Work out the finished part from the listing and answer in its coordinate system (mm). A direction names the side the tool comes from. Round coordinates to 2 decimals unless told otherwise and drop trailing zeros. Loops run counter-clockwise (first coordinate to the right, second up) from the corner with the lowest first, then second, coordinate; pieces in that order, holes last. Notation, with made-up numbers: (49, 61.25) -> (92, 61.25) arc R24 ccw to (92, 71.25) -> close; hole circle Ø6 at (42.25, 78). An arc over 180 degrees is marked (long way). Use CSV: the item, a comma, the result in double quotes. Start each with the question number.
from build123d import *

# Parameters (mm, degrees)
F0_R     = 45
F1_DEPTH = 8
F2_R     = 5
F3_W     = 23
F3_H     = 12.6
F4_DEPTH = 16.5
F5_T     = 2.5


with BuildPart() as f1:
    # F0 (on Top) → F1 (new body)
    with BuildSketch(Plane.XY):
        Circle(F0_R)
    extrude(amount=F1_DEPTH)

    # F2
    f2_edges = [f1.edges().sort_by_distance(p)[0] for p in [
        (-45, 0, 8),
    ]]
    fillet(f2_edges, radius=F2_R)

    # F3 (on Top) → F4 (join)
    with BuildSketch(Plane.XY):
        Rectangle(F3_W, F3_H)
    extrude(amount=F4_DEPTH)

    # F5
    f5_openings = [f1.faces().sort_by_distance(p)[0] for p in [
        (0, 0, 16.5),
    ]]
    offset(amount=F5_T, openings=f5_openings, kind=Kind.INTERSECTION)


solid = f1.part
Q1. For a pull along X with two mould halves and no side action, classify faces 6 (the flat face through (0, 8.8, 13)), 7 (the flat face through (11.5, 0, 12)), 8 (the flat face through (-1, 1, 0)), 9 (the cylindrical face through (-10.3, -46.37, 0.21)) as pulls with the +X half, pulls with the -X half, needs draft (parallel to the pull), parting line crosses it, or undercut.
Q2. Each of these flat-tipped pins is pushed along its axis until it touches: pin 1 (10 mm diameter, centred on x = 36, y = 10.5, fed in from +Z); pin 2 (5 mm diameter, centred on x = -5, z = 14, fed in from -Y); pin 3 (7 mm diameter, centred on y = 1.5, z = 12.5, fed in from -X). Where does it stop, or does it pass through?
Q3. Straight lines are drawn through the part: line 1 (Z direction, x = -38, y = -5); line 2 (Y direction, x = 9, z = 11.25); line 3 (Y direction, x = 0, z = 1.9). For each, find the intervals that lie inside material, in ascending order. Write a range as from..to.
Q4. Section A-A, the plane y = 0 is taken. Write down the section's boundary in (x, z).
Q5. Section C-C, the plane z = 1.75 is taken. Write down the section's boundary in (x, y), and give its area (3 significant figures).
Q6. Which of the six approach directions +Z, -Z, +X, -X, +Y, -Y give full straight-line access (tool end or side, diameter ignored) to faces 1 (the flat face through (-1, -8, 8)), 2 (the flat face through (-11.5, 0, 12)), 3 (the flat face through (-14, 0, 13)), 4 (the flat face through (14, 0, 13)), 5 (the flat face through (0, -8.8, 13))?
Q7. Section B-B, the plane x = 0 is taken. Write down the section's boundary in (y, z), and give its area (3 significant figures).
Report:
1,face 6,"needs draft"
1,face 7,"undercut"
1,face 8,"undercut"
1,face 9,"parting line crosses it"
2,pin 1,"stops at z = 10.5"
2,pin 2,"stops at y = -8.8"
2,pin 3,"stops at x = -44.48"
3,line 1,"z = -2.5..0, 8..10.5"
3,line 2,"y = -8.8..-6.3, 6.3..8.8"
3,line 3,"y = -47.5..-45, 45..47.5"
4,outline,"(-47.5, -2.5) -> (47.5, -2.5) -> (47.5, 3) arc R7.5 ccw to (40, 10.5) -> (14, 10.5) -> (14, 16.5) -> (11.5, 16.5) -> (11.5, 8) -> (40, 8) arc R5 cw to (45, 3) -> (45, 0) -> (-45, 0) -> (-45, 3) arc R5 cw to (-40, 8) -> (-11.5, 8) -> (-11.5, 16.5) -> (-14, 16.5) -> (-14, 10.5) -> (-40, 10.5) arc R7.5 ccw to (-47.5, 3) -> close"
5,outline,"circle Ø95 at (0, 0); hole circle Ø90 at (0, 0)"
5,area,"726 mm²"
6,face 1,"none"
6,face 2,"+Z"
6,face 3,"+Z, -X, +Y, -Y"
6,face 4,"+Z, +X, +Y, -Y"
6,face 5,"+Z, +X, -X, -Y"
7,outline,"(-47.5, -2.5) -> (47.5, -2.5) -> (47.5, 3) arc R7.5 ccw to (40, 10.5) -> (8.8, 10.5) -> (8.8, 16.5) -> (6.3, 16.5) -> (6.3, 8) -> (40, 8) arc R5 cw to (45, 3) -> (45, 0) -> (-45, 0) -> (-45, 3) arc R5 cw to (-40, 8) -> (-6.3, 8) -> (-6.3, 16.5) -> (-8.8, 16.5) -> (-8.8, 10.5) -> (-40, 10.5) arc R7.5 ccw to (-47.5, 3) -> close"
7,area,"500 mm²"
